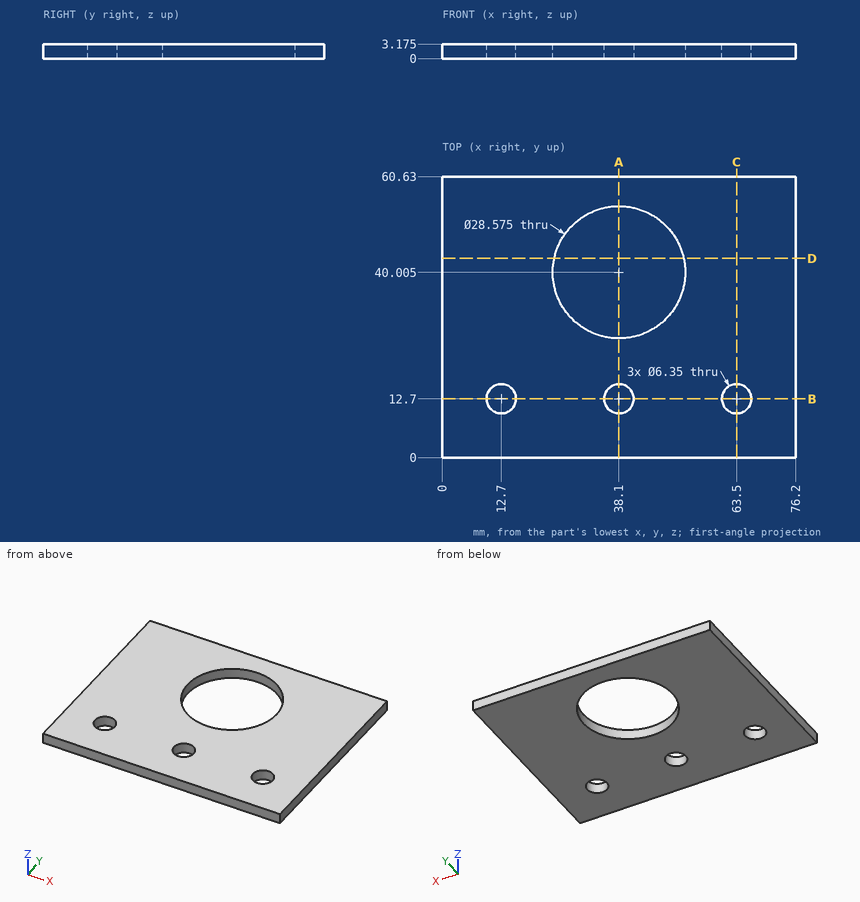
Drawing for the job (mm, zero at the part's lowest x, y, z). Give positions to 0.01 mm unless a question says otherwise; leave off trailing zeros. Loops run counter-clockwise (first coordinate to the right, second up) from the corner with the lowest first, then second, coordinate; pieces in that order, holes last.
1) Probe line 1 along Y through (x, z) = (38.1, 2.1) (1 decimal); line 2 along X through (y, z) = (15, 1.9); line 3 along Y through (x, z) = (62, 1.1). List the from-to ranges inside material, lowest first.
Values follow:
line 1: y = 0 to 9.5, 15.9 to 25.7, 54.3 to 60.6
line 2: x = 0 to 10.51, 14.89 to 35.91, 40.29 to 61.31, 65.69 to 76.2
line 3: y = 0 to 9.9, 15.5 to 60.63
2) Band-saw the part on C-C on x = 63.5. List the corners of the cut face in (y, z) (1 decimal), then the cut area to 3 significant figures.
Values follow:
outline: (0, 0) - (9.5, 0) - (9.5, 3.2) - (0, 3.2) - close; (15.9, 0) - (60.6, 0) - (60.6, 3.2) - (15.9, 3.2) - close
area: 172 mm2
3) Band-saw the part on A-A on x = 38.1. List the corners of the cut face in (y, z) (1 decimal), then the cut area to 3 significant figures.
Values follow:
outline: (0, 0) - (9.5, 0) - (9.5, 3.2) - (0, 3.2) - close; (15.9, 0) - (25.7, 0) - (25.7, 3.2) - (15.9, 3.2) - close; (54.3, 0) - (60.6, 0) - (60.6, 3.2) - (54.3, 3.2) - close
area: 81.6 mm2
4) Drop a flat-ended pin along its axis: P1, Ø23, axis at x = 38.1, y = 40.005, coming from the -Z side. Give the stop position or say it passes through.
Values follow:
P1: passes through
5) Band-saw the part on B-B on y = 12.7. List the corners of the cut face in (x, z) (3 decimals).
Values follow:
outline: (0, 0) - (9.525, 0) - (9.525, 3.175) - (0, 3.175) - close; (15.875, 0) - (34.925, 0) - (34.925, 3.175) - (15.875, 3.175) - close; (41.275, 0) - (60.325, 0) - (60.325, 3.175) - (41.275, 3.175) - close; (66.675, 0) - (76.2, 0) - (76.2, 3.175) - (66.675, 3.175) - close
6) Band-saw the part on D-D on y = 43. List the corners of the cut face in (x, z) (3 decimals).
Values follow:
outline: (0, 0) - (24.13, 0) - (24.13, 3.175) - (0, 3.175) - close; (52.07, 0) - (76.2, 0) - (76.2, 3.175) - (52.07, 3.175) - close
